```python
from build123d import *

# Parameters (mm, degrees)
EXTRUDE_1_DEPTH   = 10
EXTRUDE_1_2_DEPTH = 10
SKETCH_1_3_R      = 6
SKETCH_1_3_R_2    = 11
EXTRUDE_2_DEPTH   = 20
EXTRUDE_3_DEPTH   = 15
SKETCH_1_5_R      = 24
SKETCH_1_5_R_2    = 5
SKETCH_1_5_R_3    = 7
EXTRUDE_4_DEPTH   = 25


with BuildPart() as part:
    # Sketch 1 → Extrude 1 (new body)
    with BuildSketch(Plane.XY):
        with BuildLine():
            Line((62, -88), (62, -50))
            ThreePointArc((62, -50), (58.784609691, -62), (50, -70.784609691))
            ThreePointArc((50, -70.784609691), (31.730847168, -79.014307175), (12.187732979, -83.436586413))
            ThreePointArc((12.187732979, -83.436586413), (17.041200429, -84.37997452), (20.413213913, -87.996001687))
            Line((20.413213913, -87.996001687), (40, -130))
            Line((40, -130), (110, -130))
            ThreePointArc((110, -130), (104.727922061, -117.272077939), (92, -112))
            Line((92, -112), (86, -112))
            ThreePointArc((86, -112), (69.029437252, -104.970562748), (62, -88))
        make_face()
    extrude(amount=EXTRUDE_1_DEPTH)



with BuildPart() as body_2:
    # Sketch 1 → Extrude 1 2 (new body)
    with BuildSketch(Plane.XY):
        with BuildLine():
            ThreePointArc((-50, -70.784609691), (-58.784609691, -62), (-62, -50))
            Line((-62, -50), (-62, -88))
            ThreePointArc((-62, -88), (-69.029437252, -104.970562748), (-86, -112))
            Line((-86, -112), (-92, -112))
            ThreePointArc((-92, -112), (-104.727922061, -117.272077939), (-110, -130))
            Line((-110, -130), (-40, -130))
            Line((-40, -130), (-20.413213913, -87.996001687))
            ThreePointArc((-20.413213913, -87.996001687), (-17.041200429, -84.37997452), (-12.187732979, -83.436586413))
            ThreePointArc((-12.187732979, -83.436586413), (-31.730847168, -79.014307175), (-50, -70.784609691))
        make_face()
    extrude(amount=EXTRUDE_1_2_DEPTH)


with BuildPart() as body_3:
    # Sketch 1_3 → Extrude 2 (new body)
    with BuildSketch(Plane.XY):
        with BuildLine():
            ThreePointArc((38, 0), (0, 38), (-38, 0))
            Line((-38, 0), (-38, -14.672956535))
            ThreePointArc((-38, -14.672956535), (-40.419617314, -22.540277352), (-46.842105263, -27.688183075))
            ThreePointArc((-46.842105263, -27.688183075), (-42.500910674, -26.425823384), (-38, -26))
            ThreePointArc((-38, -26), (-21.029437252, -33.029437252), (-14, -50))
            ThreePointArc((-14, -50), (-14.740639422, -55.916261107), (-16.916845457, -61.467370864))
            ThreePointArc((-16.916845457, -61.467370864), (-17.009837453, -66.065918092), (-13.307304194, -68.794751467))
            ThreePointArc((-13.307304194, -68.794751467), (0, -69.842886359), (13.307304194, -68.794751467))
            ThreePointArc((13.307304194, -68.794751467), (17.009837453, -66.065918092), (16.916845457, -61.467370864))
            ThreePointArc((16.916845457, -61.467370864), (20.035612902, -34.085201974), (46.842105263, -27.688183075))
            ThreePointArc((46.842105263, -27.688183075), (40.419617314, -22.540277352), (38, -14.672956535))
            Line((38, -14.672956535), (38, 0))
        make_face()
        with Locations((-13.519060803, -18.607390871)):
            Circle(SKETCH_1_3_R, mode=Mode.SUBTRACT)
        Circle(SKETCH_1_3_R_2, mode=Mode.SUBTRACT)
        with Locations((-21.874299875, 7.107390871)):
            Circle(SKETCH_1_3_R, mode=Mode.SUBTRACT)
        with Locations((0, 23)):
            Circle(SKETCH_1_3_R, mode=Mode.SUBTRACT)
        with Locations((13.519060803, -18.607390871)):
            Circle(SKETCH_1_3_R, mode=Mode.SUBTRACT)
        with Locations((21.874299875, 7.107390871)):
            Circle(SKETCH_1_3_R, mode=Mode.SUBTRACT)
    extrude(amount=EXTRUDE_2_DEPTH)


with BuildPart() as part_1:
    add(part.part)

    add(body_2.part)  # Extrude 3 merges body 2

    add(body_3.part)  # Extrude 3 merges body 3
    # Sketch 1_4 → Extrude 3 (add)
    with BuildSketch(Plane.XY):
        with BuildLine():
            ThreePointArc((-16.916845457, -61.467370864), (-31.493952125, -73.10132769), (-50, -70.784609691))
            ThreePointArc((-50, -70.784609691), (-31.730847168, -79.014307175), (-12.187732979, -83.436586413))
            ThreePointArc((-12.187732979, -83.436586413), (0, -84.182069312), (12.187732979, -83.436586413))
            ThreePointArc((12.187732979, -83.436586413), (31.730847168, -79.014307175), (50, -70.784609691))
            ThreePointArc((50, -70.784609691), (31.493952125, -73.10132769), (16.916845457, -61.467370864))
            ThreePointArc((16.916845457, -61.467370864), (17.009837453, -66.065918092), (13.307304194, -68.794751467))
            ThreePointArc((13.307304194, -68.794751467), (0, -69.842886359), (-13.307304194, -68.794751467))
            ThreePointArc((-13.307304194, -68.794751467), (-17.009837453, -66.065918092), (-16.916845457, -61.467370864))
        make_face()
    extrude(amount=EXTRUDE_3_DEPTH)

    # Sketch 1_5 → Extrude 4 (add)
    # profile 1 of 2: a face of its own
    with BuildSketch(Plane.XY):
        with Locations((38, -50)):
            Circle(SKETCH_1_5_R)
        with Locations((22, -50)):
            Circle(SKETCH_1_5_R_2, mode=Mode.SUBTRACT)
        with Locations((46, -36.143593539)):
            Circle(SKETCH_1_5_R_2, mode=Mode.SUBTRACT)
        with Locations((46, -63.856406461)):
            Circle(SKETCH_1_5_R_2, mode=Mode.SUBTRACT)
        with Locations((38, -50)):
            Circle(SKETCH_1_5_R_3, mode=Mode.SUBTRACT)
    # profile 2 of 2: a face of its own
    with BuildSketch(Plane.XY):
        with Locations(Location((-38, -50, 0), (0, 0, 180))):
            Circle(SKETCH_1_5_R)
        with Locations((-46, -63.856406461)):
            Circle(SKETCH_1_5_R_2, mode=Mode.SUBTRACT)
        with Locations((-38, -50)):
            Circle(SKETCH_1_5_R_3, mode=Mode.SUBTRACT)
        with Locations((-22, -50)):
            Circle(SKETCH_1_5_R_2, mode=Mode.SUBTRACT)
        with Locations((-46, -36.143593539)):
            Circle(SKETCH_1_5_R_2, mode=Mode.SUBTRACT)
    extrude(amount=EXTRUDE_4_DEPTH)


solid = part_1.part
```
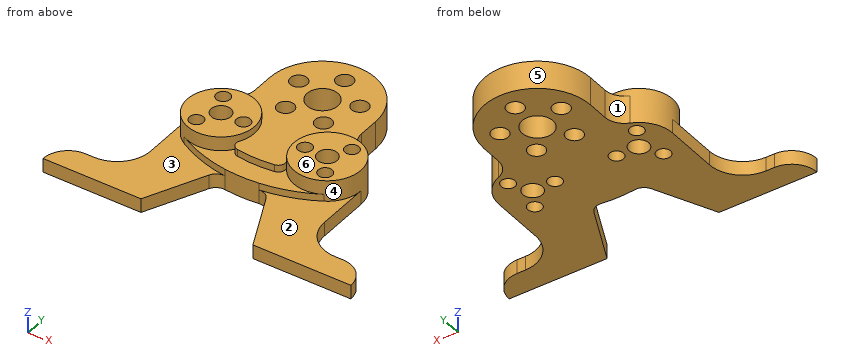
Design review of the part built by this model. Coordinates are the model's own, in mm. Face numbers are marked on the shaded views. A direction names the side the tool comes from. Coordinates: 2 decimals unless noted, no trailing zeros. Order: outer loops, then holes, each group sorted by start corner. A loop starts at its lowest first (then second) coordinate and runs counter-clockwise, first axis right, second up.
1) Mouldability with a two-part tool opening along X and no side actions: class the marked faces 4, 5 and 6 as +X half, -X half, draft (parallel to the pull), parting line (faces both ways), or undercut.
2) Take a section at D-D, the plane x = 23. Give the boundary of the cut face in (y, z) (3 decimals).
3) Take a section at A-A, the plane x = 0. Give the boundary of the cut face in (y, z).
4) Clearance check with flat-ended pins moving along their axes: pin 1 (9.5 mm diameter, centred on x = 13.52, y = -18.61, fed in from -Z); pin 2 (3 mm diameter, centred on y = -70.5, z = 4, fed in from +X); pin 3 (3 mm diameter, centred on y = -37.5, z = 4, fed in from +X); pin 4 (1 mm diameter, centred on y = -90, z = 6.5, fed in from +X). State where each tip first meets the part, or that it passes through.
5) For the marked faces 1, 2 and 3, list the 3-axis set-ups (+Z, -Z, +X, -X, +Y, -Y) from which the entire face can be reached by the end or side of a thin tool; tool diameter is ignored.
6) Wall thickness on line 1 along Y through (x, z) = (-46, 11.75); line 2 along X through (y, z) = (-51, 1.75); line 3 along X through (y, z) = (-83, 1.25): over which ranges is each line inside the solid? List them lowest first.
7) Take a section at B-B, the plane z = 22.25. State how many separate pieces and enclosed holes the cut face has, and give its area (3 significant figures).
Returned:
1. face 4: undercut
1. face 5: parting line
1. face 6: draft
2. outline: (-93.543, 0) - (-54.899, 0) - (-54.899, 25) - (-68.735, 25) - (-68.735, 15) - (-81.501, 15) - (-81.501, 10) - (-93.543, 10) - close; (-45.101, 0) - (1.214, 0) - (1.214, 20) - (-31.265, 20) - (-31.265, 25) - (-45.101, 25) - close; (13.001, 0) - (30.249, 0) - (30.249, 20) - (13.001, 20) - close
3. outline: (-84.18, 0) - (-11, 0) - (-11, 20) - (-69.84, 20) - (-69.84, 15) - (-84.18, 15) - close; (11, 0) - (17, 0) - (17, 20) - (11, 20) - close; (29, 0) - (38, 0) - (38, 20) - (29, 20) - close
4. pin 1: passes through
4. pin 2: stops at x = 62
4. pin 3: stops at x = 59.33
4. pin 4: stops at x = 62.13
5. face 1: +Z, -Z, -X, +Y
5. face 2: +Z, +X, -Y
5. face 3: +Z, -X, -Y
6. line 1: y = -72.97 to -68.86, -58.86 to -41.14, -31.14 to -27.32
6. line 2: x = -62 to -44.93, -31.07 to -26.9, -17.1 to 17.1, 26.9 to 31.07, 44.93 to 62
6. line 3: x = -62 to 62
7. separate pieces: 2
7. enclosed holes: 8
7. area: 2,840 mm2
